```python
from build123d import *

# Parameters (mm, degrees)
F0_W           = 23.846153
F0_H           = 25.673076
F0_R           = 1.772989
F0_R_2         = 5.857696
F0_R_3         = 1.386751
F0_R_4         = 1.346154
F1_DEPTH       = 4
F2_W           = 4
F2_H           = 6
F3_DEPTH       = 10
F3_FACE_W      = 4
F3_FACE_H      = 6
F4_DEPTH       = 2
F5_W           = 6
F5_H           = 6
F6_DEPTH       = 20
F8_D           = 4
F8_CSINK_D     = 6
F8_CSINK_ANGLE = 90
F9_D           = 4
F9_CSINK_D     = 6
F9_CSINK_ANGLE = 90


with BuildPart() as f1:
    # F0 (on Right) → F1 (new body)
    with BuildSketch(Plane.YZ):
        with Locations((0.673076, -12.836538)):
            Rectangle(F0_W, F0_H)
        with Locations((-6.826923, -22.403846)):
            Circle(F0_R, mode=Mode.SUBTRACT)
        with Locations((8.173076, -22.211537)):
            Circle(F0_R, mode=Mode.SUBTRACT)
        with Locations((0, -12.836538)):
            Circle(F0_R_2, mode=Mode.SUBTRACT)
        with Locations((-6.25, -2.211538)):
            Circle(F0_R_3, mode=Mode.SUBTRACT)
        with Locations((7.596153, -2.403846)):
            Circle(F0_R_4, mode=Mode.SUBTRACT)
    extrude(amount=F1_DEPTH)

    # F2 (on face) → F3 (join)
    with BuildSketch(Plane.XY):
        with Locations((2, 9.596153)):
            Rectangle(F2_W, F2_H)
        with Locations((2, -8.25)):
            Rectangle(F2_W, F2_H)
    extrude(amount=F3_DEPTH)

    # F3_face (on face) → F4 (join)
    with BuildSketch(Plane(origin=(2, 9.596153, 10), x_dir=(1, 0, 0), z_dir=(0, 0, 1))):
        Rectangle(F3_FACE_W, F3_FACE_H)
        with Locations((0, -17.846153)):
            Rectangle(F3_FACE_W, F3_FACE_H)
    extrude(amount=F4_DEPTH)

    # F5 (on face) → F6 (join)
    with BuildSketch(Plane(origin=(0, 0, 0), x_dir=(0, -1, 0), z_dir=(-1, 0, 0))):
        with Locations((-9.596153, 9)):
            Rectangle(F5_W, F5_H)
        with Locations((8.25, 9)):
            Rectangle(F5_W, F5_H)
    extrude(amount=F6_DEPTH)

    # F8 (through all)
    with Locations(Plane(origin=(0, 0, 6), x_dir=(1, 0, 0), z_dir=(0, 0, -1))):
        with Locations((-15.495499, 8.25)):
            CounterSinkHole(F8_D / 2, F8_CSINK_D / 2, counter_sink_angle=F8_CSINK_ANGLE)

    # F9 (through all)
    with Locations(Plane(origin=(0, 0, 6), x_dir=(1, 0, 0), z_dir=(0, 0, -1))):
        with Locations((-15.059971, -9.678768)):
            CounterSinkHole(F9_D / 2, F9_CSINK_D / 2, counter_sink_angle=F9_CSINK_ANGLE)


solid = f1.part
```
Work out the finished part from the listing and answer in its coordinate system (mm). A direction names the side the tool comes from. Round coordinates to 2 decimals unless told otherwise and drop trailing zeros. Write each loop counter-clockwise with the first axis right and the second up, starting at its lowest first coordinate (ties: lowest second). Pieces come first, ordered by that corner, then holes.
1) Which of the six approach directions +Z, -Z, +X, -X, +Y, -Y give full straight-line access (tool end or side, diameter ignored) to faces 4 (the face through (2, 1, 0)), 5 (the face through (-20, -8, 9)), 6 (the face through (0, 0.5, -6.5))?
2) A cutting plane is placed at A-A on z = 5. Determine the outline of the cut face in (x, y).
3) A cutting plane is placed at D-D on y = 8.25. Give the number of separate pieces and of enclosed holes in the cut face, and give its area (3 significant figures).
4) Determine the mould class of faces 1 (the face through (-19, -8, 6)), 2 (the face through (-5, 12.596, 9)), 3 (the face through (1.972, 8.991, -23.784)) for opening direction Y: pulls with the +Y half, pulls with the -Y half, needs draft (parallel to the pull), parting line crosses it, or undercut.
5) A cutting plane is placed at B-B on x = -7. Determine the outline of the cut face in (y, z), and give its area (3 significant figures).
6) Flat-ended cylindrical pins translate along their axes: P1, Ø3, axis at x = -4, y = -7, coming from the -Z side; P2, Ø12, axis at y = 5, z = -10.5, coming from the -X side; P3, Ø2, axis at x = 2.5, y = 3.5, coming from the +Z side. Find the tip coordinate at first contact, or state that the pin passes through.
7) A cutting plane is placed at C-C on z = -23. Determine the outline of the cut face in (x, y).
8) Consider probe 1 along X at (y, z) = (-8.25, 9.45); probe 2 along X at (y, z) = (8.25, -12.5); probe 3 along Z at (x, y) = (0.25, 3.25). Determine where each line is inside the solid, lowest interval first.
Entries:
1. face 4: +Z, +X, -X
1. face 5: +Z, -Z, -X, +Y, -Y
1. face 6: -Z, -X, +Y, -Y
2. outline: (0, -11.25) - (4, -11.25) - (4, -5.25) - (0, -5.25) - close; (0, 6.6) - (4, 6.6) - (4, 12.6) - (0, 12.6) - close
3. separate pieces: 4
3. enclosed holes: 0
3. area: 229 mm2
4. face 1: needs draft
4. face 2: pulls with the +Y half
4. face 3: undercut
5. outline: (-11.25, 6) - (-5.25, 6) - (-5.25, 12) - (-11.25, 12) - close; (6.6, 6) - (12.6, 6) - (12.6, 12) - (6.6, 12) - close
5. area: 72.0 mm2
6. P1: stops at z = 6
6. P2: stops at x = 0
6. P3: stops at z = 0
7. outline: (0, -11.25) - (4, -11.25) - (4, -8.5) - (0, -8.5) - close; (0, -5.16) - (4, -5.16) - (4, 6.59) - (0, 6.59) - close; (0, 9.76) - (4, 9.76) - (4, 12.6) - (0, 12.6) - close
8. probe 1: x = -20 to -17.5, -13.5 to 4
8. probe 2: x = 0 to 4
8. probe 3: z = -25.67 to -17.71, -7.96 to 0
